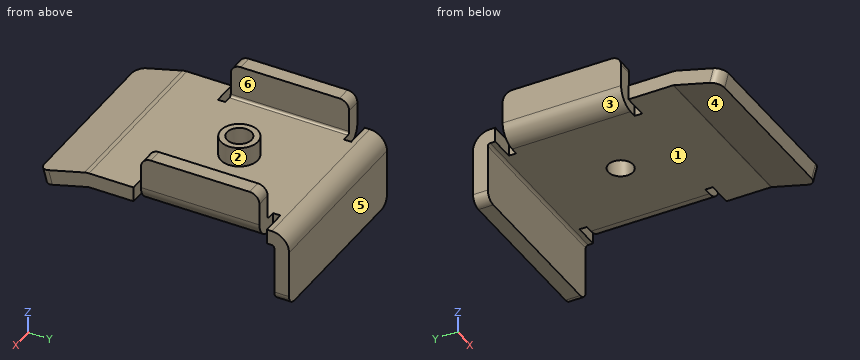
```python
from build123d import *

# Parameters (mm, degrees)
SM_BASE_FLANGE_1_DEPTH            = 18
SM_EDGE_FLANGE_1_STRIP_W          = 13
SM_EDGE_FLANGE_1_STRIP_H          = 3
SM_EDGE_FLANGE_1_STRIP_CUT_DEPTH  = 24
SM_EDGE_FLANGE_1_RELIEF_W         = 14.5
SM_EDGE_FLANGE_1_RELIEF_H         = 1.5
SM_EDGE_FLANGE_1_RELIEF_CUT_DEPTH = 3
SM_EDGE_FLANGE_1_DEPTH            = 24
SM_EDGE_FLANGE_2_STRIP_W          = 13
SM_EDGE_FLANGE_2_STRIP_H          = 3
SM_EDGE_FLANGE_2_STRIP_CUT_DEPTH  = 24
SM_EDGE_FLANGE_2_RELIEF_W         = 14.5
SM_EDGE_FLANGE_2_RELIEF_H         = 1.5
SM_EDGE_FLANGE_2_RELIEF_CUT_DEPTH = 3
SM_EDGE_FLANGE_2_DEPTH            = 24
SKETCH_12_R                       = 3.75
EXTRUDE_1_DEPTH                   = 7
HOLE_WIZARD_M6_1_D                = 5
HOLE_WIZARD_M6_1_DEPTH            = 15
HOLE_WIZARD_M6_1_TIP              = 1.502151548
FILLET_1_R                        = 2


# Sheet-metal steps are written as plain solids
with BuildPart() as part:
    # 草图2 → 基体-法兰1 (new, symmetric)
    with BuildSketch(Plane(origin=(0, 0, 0), x_dir=(0, 0, -1), z_dir=(1, 0, 0))):
        with BuildLine():
            Line((2.588190451, -9.659258263), (0.119259608, -0.445082916))
            ThreePointArc((0.119259608, -0.445082916), (0.029942985, 0.003942069), (0, 0.460783742))
            Line((0, 0.460783742), (0, 37.5))
            ThreePointArc((0, 37.5), (1.025126266, 39.974873734), (3.5, 41))
            Line((3.5, 41), (15, 41))
            Line((15, 41), (15, 38))
            Line((15, 38), (3.5, 38))
            ThreePointArc((3.5, 38), (3.146446609, 37.853553391), (3, 37.5))
            Line((3, 37.5), (3, 0.460783742))
            ThreePointArc((3, 0.460783742), (3.004277569, 0.395520645), (3.017037087, 0.331374219))
            Line((3.017037087, 0.331374219), (5.48596793, -8.882801128))
            Line((5.48596793, -8.882801128), (2.588190451, -9.659258263))
        make_face()
    extrude(amount=SM_BASE_FLANGE_1_DEPTH, both=True)

    # 边线-法兰1 strip (across the edge) → 边线-法兰1 strip cut (cut)
    with BuildSketch(Plane(origin=(18, 11, 0), x_dir=(-1, 0, 0), z_dir=(0, 1, 0))):
        with Locations((-3, -1.5)):
            Rectangle(SM_EDGE_FLANGE_1_STRIP_W, SM_EDGE_FLANGE_1_STRIP_H)
    extrude(amount=SM_EDGE_FLANGE_1_STRIP_CUT_DEPTH, mode=Mode.SUBTRACT)

    # 边线-法兰1 relief (on the sheet) → 边线-法兰1 relief cut (cut)
    with BuildSketch(Plane(origin=(14.5, 11, 0), x_dir=(-1, 0, 0), z_dir=(0, 0, 1))):
        with Locations((-5.75, 0.75)):
            Rectangle(SM_EDGE_FLANGE_1_RELIEF_W, SM_EDGE_FLANGE_1_RELIEF_H)
        with Locations((-5.75, -24.75)):
            Rectangle(SM_EDGE_FLANGE_1_RELIEF_W, SM_EDGE_FLANGE_1_RELIEF_H)
    extrude(amount=-SM_EDGE_FLANGE_1_RELIEF_CUT_DEPTH, mode=Mode.SUBTRACT)

    # 边线-法兰1 section (across the edge) → 边线-法兰1 (add)
    with BuildSketch(Plane(origin=(18, 11, 0), x_dir=(-1, 0, 0), z_dir=(0, 1, 0))):
        with BuildLine():
            Line((0, 0.5), (0, 7))
            Line((0, 7), (3, 7))
            Line((3, 7), (3, 0.5))
            ThreePointArc((3, 0.5), (3.146446609, 0.146446609), (3.5, 0))
            Line((3.5, 0), (3.5, -3))
            ThreePointArc((3.5, -3), (1.025126266, -1.974873734), (0, 0.5))
        make_face()
    extrude(amount=SM_EDGE_FLANGE_1_DEPTH)

    # 边线-法兰2 strip (across the edge) → 边线-法兰2 strip cut (cut)
    with BuildSketch(Plane(origin=(-18, 35, 0), x_dir=(1, 0, 0), z_dir=(0, -1, 0))):
        with Locations((-3, -1.5)):
            Rectangle(SM_EDGE_FLANGE_2_STRIP_W, SM_EDGE_FLANGE_2_STRIP_H)
    extrude(amount=SM_EDGE_FLANGE_2_STRIP_CUT_DEPTH, mode=Mode.SUBTRACT)

    # 边线-法兰2 relief (on the sheet) → 边线-法兰2 relief cut (cut)
    with BuildSketch(Plane(origin=(-14.5, 35, 0), x_dir=(1, 0, 0), z_dir=(0, 0, 1))):
        with Locations((-5.75, 0.75)):
            Rectangle(SM_EDGE_FLANGE_2_RELIEF_W, SM_EDGE_FLANGE_2_RELIEF_H)
        with Locations((-5.75, -24.75)):
            Rectangle(SM_EDGE_FLANGE_2_RELIEF_W, SM_EDGE_FLANGE_2_RELIEF_H)
    extrude(amount=-SM_EDGE_FLANGE_2_RELIEF_CUT_DEPTH, mode=Mode.SUBTRACT)

    # 边线-法兰2 section (across the edge) → 边线-法兰2 (add)
    with BuildSketch(Plane(origin=(-18, 35, 0), x_dir=(1, 0, 0), z_dir=(0, -1, 0))):
        with BuildLine():
            Line((0, 0.5), (0, 7))
            Line((0, 7), (3, 7))
            Line((3, 7), (3, 0.5))
            ThreePointArc((3, 0.5), (3.146446609, 0.146446609), (3.5, 0))
            Line((3.5, 0), (3.5, -3))
            ThreePointArc((3.5, -3), (1.025126266, -1.974873734), (0, 0.5))
        make_face()
    extrude(amount=SM_EDGE_FLANGE_2_DEPTH)

    # 草图12 → 凸台-拉伸1 (add)
    with BuildSketch(Plane(origin=(0, 0, -3), x_dir=(-1, 0, 0), z_dir=(0, 0, -1))):
        with Locations((0, 21)):
            Circle(SKETCH_12_R)
    extrude(amount=-EXTRUDE_1_DEPTH)

    # M6 螺纹孔1
    with Locations(Plane(origin=(0, 0, -3), x_dir=(-1, 0, 0), z_dir=(0, 0, -1))):
        with Locations((0, 21)):
            Hole(HOLE_WIZARD_M6_1_D / 2, depth=HOLE_WIZARD_M6_1_DEPTH)
            with Locations((0, 0, -(HOLE_WIZARD_M6_1_DEPTH + HOLE_WIZARD_M6_1_TIP / 2))):  # 118° drill point
                Cone(0, HOLE_WIZARD_M6_1_D / 2, HOLE_WIZARD_M6_1_TIP, mode=Mode.SUBTRACT)

    # 圆角1
    fillet_1_edges = [part.edges().sort_by_distance(p)[0] for p in [
        (-18, -9.271029695, -4.03707919),
        (-16.5, 35, 7),
        (-16.5, 11, 7),
        (-18, 39.5, -15),
        (18, -9.271029695, -4.03707919),
        (18, 39.5, -15),
        (16.5, 11, 7),
        (16.5, 35, 7),
    ]]
    fillet(fillet_1_edges, radius=FILLET_1_R)


solid = part.part
```
Source: CAD feature listing. Evaluate the final solid. Frame: model axes, mm. Face numbers are marked on the shaded views. A direction names the side the tool comes from. Give positions to 0.01 mm unless a question says otherwise; leave off trailing zeros. Loops run counter-clockwise (first coordinate to the right, second up) from the corner with the lowest first, then second, coordinate; pieces in that order, holes last. Notation, with made-up numbers: (70, 24.5) -> (110, 24.5) arc R20 cw to (110, 38.5) -> close; hole circle Ø9 at (76, -22). An arc over 180 degrees is marked (long way). Put each result on its own line as item: value. Start each with the question number.
1) Cut plane B-B (y = 21). Return loops of the section in (x, z), then the cut area to 3 significant figures.
2) Reachability of the marked faces 1, 2 and 3 from +Z, -Z, +X, -X, +Y, -Y: full face, straight path, thin tool, end or side. Return the list, or none.
3) Cut plane D-D (y = 8). Return loops of the section in (x, z).
4) Draft query along Y for the marked faces 4, 5 and 6. Return one class per face: released by +Y, released by -Y, zero draft, split by the parting line, or undercut.
5) Cut plane C-C (x = 9.5). Return loops of the section in (y, z).
6) Cut plane A-A (x = 0). Return loops of the section in (y, z), then the cut area to 3 significant figures.
7) Material intervals for probe 1 along X at (y, z) = (11.5, 4); probe 2 along Y at (x, z) = (0, 0.75); probe 3 along Y at (x, z) = (13.5, -7), sorted ascending.
8) Contact query for flat-ended pins moving along their axis: P1, Ø1.6, axis at y = 35.5, z = -1.5, coming from the +X side; P2, Ø6, axis at x = -3, z = -6.5, coming from the -Y side; P3, Ø2.5, axis at x = 14.5, z = -1, coming from the +Y side; P4, Ø6, axis at x = -10.5, z = 4.5, coming from the +Y side. Output: stop coordinate, or through.
Results are:
1. outline: (-18, 0.5) arc R3.5 ccw to (-14.5, -3) -> (-2.5, -3) -> (-2.5, 4) -> (-3.75, 4) -> (-3.75, 0) -> (-14.5, 0) arc R0.5 cw to (-15, 0.5) -> (-15, 7) -> (-18, 7) -> close; (2.5, -3) -> (14.5, -3) arc R3.5 ccw to (18, 0.5) -> (18, 7) -> (15, 7) -> (15, 0.5) arc R0.5 cw to (14.5, 0) -> (3.75, 0) -> (3.75, 4) -> (2.5, 4) -> close
1. area: 140 mm2
2. face 1: -Z, +X, -X
2. face 2: +Z
2. face 3: -Z, -X
3. outline: (-18, -3) -> (18, -3) -> (18, 0) -> (-18, 0) -> close
4. face 4: undercut
4. face 5: released by +Y
4. face 6: zero draft
5. outline: (-9.66, -2.59) -> (-8.88, -5.49) -> (0.33, -3.02) arc R0.5 cw to (0.46, -3) -> (37.5, -3) arc R0.5 cw to (38, -3.5) -> (38, -15) -> (41, -15) -> (41, -3.5) arc R3.5 ccw to (37.5, 0) -> (0.46, 0) arc R3.5 ccw to (-0.45, -0.12) -> close
6. outline: (-9.66, -2.59) -> (-8.88, -5.49) -> (0.33, -3.02) arc R0.5 cw to (0.46, -3) -> (18.5, -3) -> (18.5, 4) -> (17.25, 4) -> (17.25, 0) -> (0.46, 0) arc R3.5 ccw to (-0.45, -0.12) -> close; (23.5, -3) -> (37.5, -3) arc R0.5 cw to (38, -3.5) -> (38, -15) -> (41, -15) -> (41, -3.5) arc R3.5 ccw to (37.5, 0) -> (24.75, 0) -> (24.75, 4) -> (23.5, 4) -> close
6. area: 180 mm2
7. probe 1: x = -18 to -15, 15 to 18
7. probe 2: y = 17.25 to 18.5, 23.5 to 24.75
7. probe 3: y = 38 to 41
8. P1: stops at x = 17.72
8. P2: stops at y = -9.41
8. P3: stops at y = 40.77
8. P4: passes through
